CAD build for the part. Positions are in the model's coordinates, mm. Face numbers are marked on the shaded views. A direction names the side the tool comes from. Coordinates: 2 decimals unless noted, no trailing zeros. Loops run counter-clockwise (first coordinate to the right, second up) from the corner with the lowest first, then second, coordinate; pieces in that order, holes last. Notation, with made-up numbers: (-8, 33.25) -> (8, 33.25) arc R16 cw to (8, 39.25) -> close; hole circle Ø8 at (-13, 16). An arc over 180 degrees is marked (long way). Answer as CSV lines item,"result". Start each with the question number.
from build123d import *

# Parameters (mm, degrees)
CORTAR_EXTRUIR1_DEPTH      = 34.678925161
CORTAR_EXTRUIR1_DEPTH_BACK = 34.678925161
CROQUIS5_R                 = 3
CORTAR_EXTRUIR3_DEPTH      = 22
REDONDEO5_R                = 0.3
CHAFL_N1_SIZE              = 0.145725928


with BuildPart() as part:
    # Croquis1 → Revolución1 (revolve)
    with BuildSketch(Plane.XY):
        with BuildLine():
            Line((-5, -8.775534172), (-5, -24.775534172))
            Line((-5, -24.775534172), (-6.5, -26.638122331))
            Line((-6.5, -26.638122331), (-6.5, -30.5))
            Line((-6.5, -30.5), (0, -30.5))
            Line((0, -30.5), (0, -6.4))
            ThreePointArc((0, -6.4), (-6.4, 0), (0, 6.4))
            Line((0, 6.4), (0, 10.1))
            ThreePointArc((0, 10.1), (-9.763270332, 2.586223585), (-5, -8.775534172))
        make_face()
    revolve(axis=Axis((0, -6.4, 0), (0, -1, 0)))

    # Croquis2 → Cortar-Extruir1 (cut, two sides: drawn at the far end of the back side and taken through both)
    with BuildSketch(Plane.XY.offset(-CORTAR_EXTRUIR1_DEPTH_BACK)):
        Polygon((6.3, -11.775534172), (3.3, -8.775534172), (3.3, 15.005915622), (11.326938796, 15.005915622), (10.720239286, -11.775534172), align=None)
        Polygon((-3.3, -8.775534172), (-3.3, 15.005915622), (-11.844039482, 15.005915622), (-11.844039482, -11.775534172), (-6.3, -11.775534172), align=None)
    extrude(amount=CORTAR_EXTRUIR1_DEPTH + CORTAR_EXTRUIR1_DEPTH_BACK, mode=Mode.SUBTRACT)

    # Croquis5 → Cortar-Extruir3 (cut)
    with BuildSketch(Plane.XZ.offset(30.5)):
        Circle(CROQUIS5_R)
    extrude(amount=-CORTAR_EXTRUIR3_DEPTH, mode=Mode.SUBTRACT)

    # Redondeo5
    redondeo5_edges = [part.edges().sort_by_distance(p)[0] for p in [
        (-3, -30.5, 0),
    ]]
    fillet(redondeo5_edges, radius=REDONDEO5_R)

    # Chaflán1
    # the kernel refuses this chamfer: 0.2, 0.145725928 mm, written as the material it takes off along each edge
    with BuildSketch(Plane(origin=(3.3, 0, 0), x_dir=(0, 0, -1), z_dir=(0, 1, 0))) as chafl_n1_piece_1:
        with BuildLine():
            Line((5.483611948 + CHAFL_N1_SIZE * 0.999999998153, 0), (5.585635764, 0.175792403))
            ThreePointArc((5.585635764, 0.175792403), (5.536764117, 0.089977708), (5.483611948, 0))
            Line((5.483611948, 0), (5.483611948 + CHAFL_N1_SIZE * 0.999999998153, 0))
        make_face()
    revolve(axis=Axis((3.3, 0, 0), (-1, 0, 0)), mode=Mode.SUBTRACT)
    with BuildSketch(Plane(origin=(-3.3, 0, 0), x_dir=(0, 1, 0), z_dir=(0, 0, 1))) as chafl_n1_piece_2:
        with BuildLine():
            Line((5.483611948 + CHAFL_N1_SIZE * 0.999999998153, 0), (5.585635764, -0.175792403))
            ThreePointArc((5.585635764, -0.175792403), (5.536764117, -0.089977708), (5.483611948, 0))
            Line((5.483611948, 0), (5.483611948 + CHAFL_N1_SIZE * 0.999999998153, 0))
        make_face()
    revolve(axis=Axis((-3.3, 0, 0), (-1, 0, 0)), revolution_arc=180, mode=Mode.SUBTRACT)
    with BuildSketch(Plane(origin=(-3.3, 0, 0), x_dir=(0, -1, 0), z_dir=(0, 0, -1))) as chafl_n1_piece_3:
        with BuildLine():
            Line((5.483611948 + CHAFL_N1_SIZE * 0.999999998153, 0), (5.585635764, -0.175792403))
            ThreePointArc((5.585635764, -0.175792403), (5.536764117, -0.089977708), (5.483611948, 0))
            Line((5.483611948, 0), (5.483611948 + CHAFL_N1_SIZE * 0.999999998153, 0))
        make_face()
    revolve(axis=Axis((-3.3, 0, 0), (-1, 0, 0)), revolution_arc=180, mode=Mode.SUBTRACT)


solid = part.part
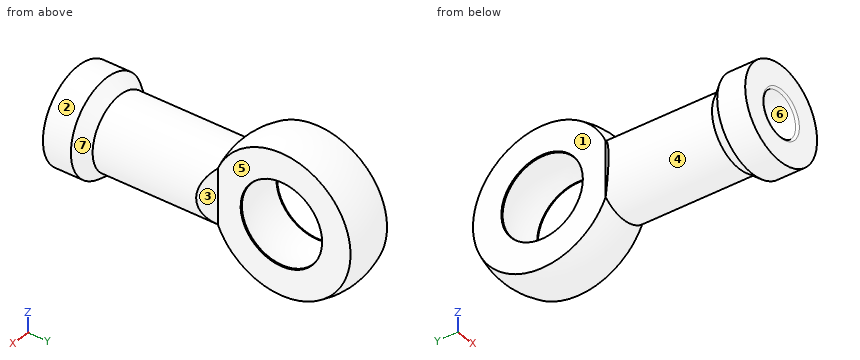
Item 1: Saw through at B-B (y = 0). Write the cut outline in (x, z), plus the area to 3 significant figures.
Item 2: Two-plate mould, pull along Z, no slides. Class the marked faces 5, 6 and 7: pulls with the +Z half, pulls with the -Z half, needs draft (parallel to the pull), parting line crosses it, or undercut.
Item 3: Saw through at C-C (z = 0). Write the cut outline in (x, y).
Item 4: Saw through at D-D (y = -7). Write the cut outline in (x, z), plus the area to 3 significant figures.
Item 5: Wall check: probe 1 along Z at (x, y) = (0, -14.25); probe 2 along Y at (x, z) = (-0.5, 5.75); probe 3 along Y at (x, z) = (-0.5, 4.5). Give the ranges that are in metal, low to high.
Item 6: Saw through at A-A (x = 0). Write the cut outline in (y, z).
Item 7: Flat gauge pins, fed straight in: pin 1 Ø2 at (y, z) = (-6.5, 7.5) entering from -X; pin 2 Ø1 at (x, z) = (-3, -8) entering from -Y; pin 3 Ø2 at (y, z) = (-16, -3.5) entering from -X. Where does each tip first touch, or does it go through?
Item 8: Which spindle directions (+Z, -Z, +X, -X, +Y, -Y) get a long thin tool onto all of the face, cutting with end or side? Do the marked faces 1, 2, 3 and 4. Say none if no direction does.
Geometry check:
1,outline,"(-3.3, -9.55) arc R10.1 ccw to (3.3, -9.55) -> (3.3, -5.63) -> (3.12, -5.59) arc R6.4 cw to (-3.12, -5.59) -> (-3.3, -5.63) -> close; (-3.3, 5.63) -> (-3.12, 5.59) arc R6.4 cw to (3.12, 5.59) -> (3.3, 5.63) -> (3.3, 9.55) arc R10.1 ccw to (-3.3, 9.55) -> close"
1,area,"50.3 mm2"
2,face 5,"needs draft"
2,face 6,"undercut"
2,face 7,"parting line crosses it"
3,outline,"(-6.5, -30.5) -> (-3.3, -30.5) arc R0.3 ccw to (-3, -30.2) -> (-3, -8.5) -> (3, -8.5) -> (3, -30.2) arc R0.3 ccw to (3.3, -30.5) -> (6.5, -30.5) -> (6.5, -26.64) -> (5, -24.78) -> (5, -10.48) -> (3.3, -8.78) -> (3.3, -5.63) -> (3.12, -5.59) arc R6.4 cw to (-3.12, -5.59) -> (-3.3, -5.63) -> (-3.3, -8.78) -> (-5, -10.48) -> (-5, -24.78) -> (-6.5, -26.64) -> close; (-3.3, 5.63) -> (-3.12, 5.59) arc R6.4 cw to (3.12, 5.59) -> (3.3, 5.63) -> (3.3, 9.55) arc R10.1 ccw to (-3.3, 9.55) -> close"
4,outline,"(-3.3, -6.49) arc R7.28 ccw to (3.3, -6.49) -> (3.3, 6.49) arc R7.28 ccw to (-3.3, 6.49) -> close"
4,area,"92.7 mm2"
5,probe 1,"-5 to -3, 3 to 5"
5,probe 2,"-30.5 to -25.73, -8.29 to -2.77, 2.77 to 8.29"
5,probe 3,"-30.5 to -4.52, 4.52 to 9.03"
6,outline,"(-30.5, -6.5) -> (-26.64, -6.5) -> (-24.78, -5) -> (-8.78, -5) arc R10.1 ccw (long way) to (-8.78, 5) -> (-24.78, 5) -> (-26.64, 6.5) -> (-30.5, 6.5) -> (-30.5, 3.3) arc R0.3 ccw to (-30.2, 3) -> (-8.5, 3) -> (-8.5, -3) -> (-30.2, -3) arc R0.3 ccw to (-30.5, -3.3) -> close; hole circle Ø12.8 at (0, 0)"
7,pin 1,"x = -3.3"
7,pin 2,"y = -6.11"
7,pin 3,"x = -4.33"
8,face 1,"+Z, -Z, -X, +Y"
8,face 2,"-Y"
8,face 3,"+Z, -Z, +X, +Y"
8,face 4,"none"
